from build123d import *

# Parameters (mm, degrees)
SUPPORT_DEPTH              = 3.5
MAIN_FEATURES_SKETCH_3_R   = 6.25
KNOB_DEPTH                 = 3.7
SHAFT_START                = -3.7
MAIN_FEATURES_SKETCH_4_R   = 1.75
SHAFT_DEPTH                = 0.9
LEGS_START                 = 3.5
MAIN_FEATURES_SKETCH_5_R   = 1
MAIN_FEATURES_SKETCH_5_R_2 = 0.5
LEGS_DEPTH                 = 2.5


with BuildPart() as part:
    # main_features_sketch → support (new body)
    with BuildSketch(Plane.XY):
        with BuildLine():
            Line((0.5, -6.9), (0.5, -1.687971711))
            Line((0.5, -1.687971711), (3.338674058, -6.059146436))
            ThreePointArc((3.338674058, -6.059146436), (4.030328859, -6.206162203), (4.177344626, -5.514507401))
            Line((4.177344626, -5.514507401), (1.332722713, -1.134173783))
            ThreePointArc((1.332722713, -1.134173783), (1.386056185, -1.068339015), (1.436140662, -1))
            Line((1.436140662, -1), (7.5, -1))
            ThreePointArc((7.5, -1), (8.5, 0), (7.5, 1))
            Line((7.5, 1), (1.436140662, 1))
            ThreePointArc((1.436140662, 1), (0, 1.75), (-1.436140662, 1))
            Line((-1.436140662, 1), (-7.5, 1))
            ThreePointArc((-7.5, 1), (-8.5, 0), (-7.5, -1))
            Line((-7.5, -1), (-1.436140662, -1))
            ThreePointArc((-1.436140662, -1), (-1.386056185, -1.068339015), (-1.332722713, -1.134173783))
            Line((-1.332722713, -1.134173783), (-4.177344626, -5.514507401))
            ThreePointArc((-4.177344626, -5.514507401), (-4.030328859, -6.206162203), (-3.338674058, -6.059146436))
            Line((-3.338674058, -6.059146436), (-0.5, -1.687971711))
            Line((-0.5, -1.687971711), (-0.5, -6.9))
            ThreePointArc((-0.5, -6.9), (0, -7.4), (0.5, -6.9))
        make_face()
    extrude(amount=SUPPORT_DEPTH)

    # main_features_sketch<3> → knob (add)
    with BuildSketch(Plane.XY):
        Circle(MAIN_FEATURES_SKETCH_3_R)
    extrude(amount=-KNOB_DEPTH)

    # main_features_sketch<4> → shaft (add)
    with BuildSketch(Plane.XY.offset(SHAFT_START)):
        Circle(MAIN_FEATURES_SKETCH_4_R)
    extrude(amount=-SHAFT_DEPTH)

    # main_features_sketch<5> → legs (add)
    with BuildSketch(Plane.XY.offset(LEGS_START)):
        with Locations(Location((-7.5, 0, 0), (0, 0, 270))):
            Circle(MAIN_FEATURES_SKETCH_5_R)
        with Locations(Location((-3.758009342, -5.786826919, 0), (0, 0, 147))):
            Circle(MAIN_FEATURES_SKETCH_5_R_2)
        with Locations((0, -6.9)):
            Circle(MAIN_FEATURES_SKETCH_5_R_2)
        with Locations(Location((3.758009342, -5.786826919, 0), (0, 0, 213))):
            Circle(MAIN_FEATURES_SKETCH_5_R_2)
        with Locations(Location((7.5, 0, 0), (0, 0, 90))):
            Circle(MAIN_FEATURES_SKETCH_5_R)
    extrude(amount=LEGS_DEPTH)


solid = part.part
The listing builds one solid part. Answer for the finished solid, in the listing's coordinates (mm). A direction names the side the tool comes from. Coordinates: 2 decimals unless noted, no trailing zeros. Loops run counter-clockwise (first coordinate to the right, second up) from the corner with the lowest first, then second, coordinate; pieces in that order, holes last. Notation, with made-up numbers: (31, 56) -> (76, 56) arc R17 cw to (76, 70) -> close; hole circle Ø6 at (19, 66). An arc over 180 degrees is marked (long way). Answer in a Markdown table with one row per item. Add a question column.
1. The part is cut by section B-B, the plane x = 0. Write down the section's boundary in (y, z), then the cut area to 3 significant figures.
2. The part is cut by section C-C, the plane z = 4.5. Write down the section's boundary in (x, y).
3. Flat-ended cylindrical pins translate along their axes: P1, Ø2.5, axis at x = -3.5, y = -0.5, coming from the +Z side; P2, Ø6, axis at y = -3.5, z = 2.5, coming from the -X side; P3, Ø1.6, axis at x = -1.5, y = 3.5, coming from the +Z side. Find the tip coordinate at first contact, or state that the pin passes through.
4. Consider line 1 (X direction, y = -5.25, z = 1.75); line 2 (Y direction, x = 6.25, z = 0.5); line 3 (X direction, y = -5.75, z = 3.25). Determine where each line is inside the solid, lowest interval first. Write a range as [from, to].
5. The part is cut by section D-D, the plane y = -2. Write down the section's boundary in (x, z) (3 decimals).
6. For faces 4 (the flat face through (-2.735, -3.294, 1.726)), 5 (the cylindrical face through (-8.498, 0.066, 2.958)), 6 (the flat face through (-4, 1, 2)), 7 (the flat face through (4, -1, 2)), 8 (the flat face through (1, -4, 0)), determine the directions among +Z, -Z, +X, -X, +Y, -Y from which every point of the face is accessible in a straight line to the end or side of a thin tool.
7. Determine the mould class of faces 1 (the flat face through (-7, 0, 0)), 2 (the cylindrical face through (0.231, -7.344, 3.625)), 3 (the flat face through (0, -2, 3.5)) for opening direction X: +X half, -X half, draft (parallel to the pull), parting line (faces both ways), or undercut.
8. The part is cut by section A-A, the plane z = 2. Write down the section's boundary in (x, y), then the cut area to 3 significant figures.
Answer below:
| question | item | result |
|---|---|---|
| 1 | outline | (-7.4, 0) -> (-6.25, 0) -> (-6.25, -3.7) -> (-1.75, -3.7) -> (-1.75, -4.6) -> (1.75, -4.6) -> (1.75, -3.7) -> (6.25, -3.7) -> (6.25, 0) -> (1.75, 0) -> (1.75, 3.5) -> (-6.4, 3.5) -> (-6.4, 6) -> (-7.4, 6) -> close |
| 1 | area | 83.9 mm2 |
| 2 | outline | circle Ø2 at (-7.5, 0); circle Ø1 at (-3.76, -5.79); circle Ø1 at (0, -6.9); circle Ø1 at (3.76, -5.79); circle Ø2 at (7.5, 0) |
| 3 | P1 | z = 3.5 |
| 3 | P2 | x = -8.37 |
| 3 | P3 | z = 0 |
| 4 | line 1 | [-4.01, -2.81], [-0.5, 0.5], [2.81, 4.01] |
| 4 | line 2 | [-1, 1] |
| 4 | line 3 | [-4.26, -3.14], [-0.5, 0.5], [3.14, 4.26] |
| 5 | outline | (-5.921, -3.7) -> (5.921, -3.7) -> (5.921, 0) -> (1.895, 0) -> (1.895, 3.5) -> (0.703, 3.5) -> (0.703, 0) -> (0.5, 0) -> (0.5, 3.5) -> (-0.5, 3.5) -> (-0.5, 0) -> (-0.703, 0) -> (-0.703, 3.5) -> (-1.895, 3.5) -> (-1.895, 0) -> (-5.921, 0) -> close |
| 6 | face 4 | +Z, -X |
| 6 | face 5 | +Z |
| 6 | face 6 | +Z, -X, +Y |
| 6 | face 7 | +Z, +X |
| 6 | face 8 | +Z, -Y |
| 7 | face 1 | draft |
| 7 | face 2 | parting line |
| 7 | face 3 | undercut |
| 8 | outline | (-7.5, -1) -> (-1.44, -1) arc R1.75 ccw to (-1.33, -1.13) -> (-4.18, -5.51) arc R0.5 ccw to (-3.34, -6.06) -> (-0.5, -1.69) -> (-0.5, -6.9) arc R0.5 ccw to (0.5, -6.9) -> (0.5, -1.69) -> (3.34, -6.06) arc R0.5 ccw to (4.18, -5.51) -> (1.33, -1.13) arc R1.75 ccw to (1.44, -1) -> (7.5, -1) arc R1 ccw to (7.5, 1) -> (1.44, 1) arc R1.75 ccw to (-1.44, 1) -> (-7.5, 1) arc R1 ccw to start |
| 8 | area | 52.9 mm2 |
